from build123d import *

# Parameters (mm, degrees)
SKETCH1_W           = 250
SKETCH1_H           = 267.4
SKETCH1_R           = 2.5
SKETCH1_W_2         = 33
SKETCH1_H_2         = 90
BOSS_EXTRUDE1_DEPTH = 5
SKETCH6_W           = 250
SKETCH6_H           = 70.024397165
CUT_EXTRUDE4_DEPTH  = 6


with BuildPart() as part:
    # Sketch1 → Boss-Extrude1 (new body)
    with BuildSketch(Plane.XY):
        with Locations((-3272.432417868, -202.7)):
            Rectangle(SKETCH1_W, SKETCH1_H)
        with Locations((-3151.432417868, -193.5)):
            Circle(SKETCH1_R, mode=Mode.SUBTRACT)
        with Locations((-3151.432417868, -244.5)):
            Circle(SKETCH1_R, mode=Mode.SUBTRACT)
        with Locations((-3393.432417868, -244.5)):
            Circle(SKETCH1_R, mode=Mode.SUBTRACT)
        with Locations((-3393.432417868, -193.5)):
            Circle(SKETCH1_R, mode=Mode.SUBTRACT)
        with Locations((-3195.572417868, -219)):
            Rectangle(SKETCH1_W_2, SKETCH1_H_2, mode=Mode.SUBTRACT)
        with Locations((-3349.292417868, -219)):
            Rectangle(SKETCH1_W_2, SKETCH1_H_2, mode=Mode.SUBTRACT)
    extrude(amount=BOSS_EXTRUDE1_DEPTH)

    # Sketch6 → Cut-Extrude4 (cut, through all)
    with BuildSketch(Plane.XY.offset(5)):
        with BuildLine():
            Line((-3243.992329325, -69), (-3147.432417868, -69))
            Line((-3147.432417868, -69), (-3147.432417868, -182))
            Line((-3147.432417868, -182), (-3174.036756226, -182))
            Line((-3174.036756226, -182), (-3174.036756226, -154))
            Line((-3174.036756226, -154), (-3185.682810376, -154))
            ThreePointArc((-3185.682810376, -154), (-3237.221630697, -126.855339059), (-3243.992329325, -69))
        make_face()
        with Locations((-3272.432417868, -301.387801417)):
            Rectangle(SKETCH6_W, SKETCH6_H)
        with BuildLine():
            Line((-3300.872506412, -69), (-3397.432417868, -69))
            Line((-3397.432417868, -69), (-3397.432417868, -182))
            Line((-3397.432417868, -182), (-3370.82807951, -182))
            Line((-3370.82807951, -182), (-3370.82807951, -154))
            Line((-3370.82807951, -154), (-3359.18202536, -154))
            ThreePointArc((-3359.18202536, -154), (-3307.64320504, -126.855339059), (-3300.872506412, -69))
        make_face()
    extrude(amount=-CUT_EXTRUDE4_DEPTH, mode=Mode.SUBTRACT)


solid = part.part
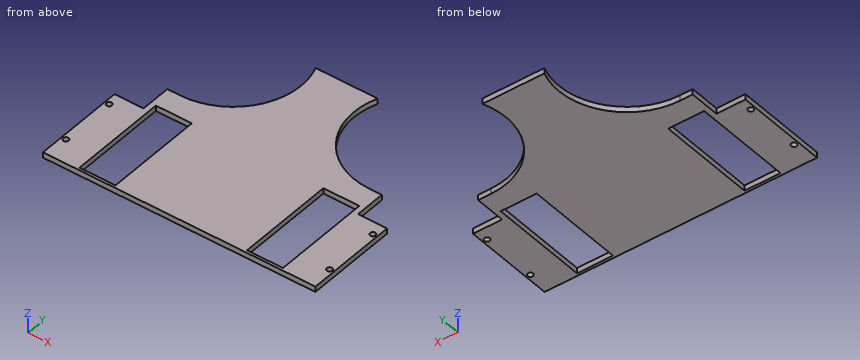
Input: part model. Units: mm. Frame: model coordinates. Round coordinates to 2 decimals unless told otherwise and drop trailing zeros. Order: outer loops, then holes, each group sorted by start corner. A loop starts at its lowest first (then second) coordinate and runs counter-clockwise, first axis right, second up.
1. Cut plane B-B, the plane z = 3.5. Output: boundary loops of the cut face in (x, y).
The answers:
outline: (-3397.43, -266.38) - (-3147.43, -266.38) - (-3147.43, -182) - (-3174.04, -182) - (-3174.04, -154) - (-3185.68, -154) arc R62.5 cw to (-3243.99, -69) - (-3300.87, -69) arc R62.5 cw to (-3359.18, -154) - (-3370.83, -154) - (-3370.83, -182) - (-3397.43, -182) - close; hole circle Ø5 at (-3393.43, -244.5); hole circle Ø5 at (-3393.43, -193.5); hole (-3365.79, -264) - (-3332.79, -264) - (-3332.79, -174) - (-3365.79, -174) - close; hole (-3212.07, -264) - (-3179.07, -264) - (-3179.07, -174) - (-3212.07, -174) - close; hole circle Ø5 at (-3151.43, -244.5); hole circle Ø5 at (-3151.43, -193.5)
2. Material intervals for line 1 (X direction, y = -178.5, z = 2.8); line 2 (X direction, y = -244.5, z = 3.7); line 3 (X direction, y = -201.5, z = 3.15), sorted ascending.
The answers:
line 1: x = -3370.83 to -3365.79, -3332.79 to -3212.07, -3179.07 to -3174.04
line 2: x = -3397.43 to -3395.93, -3390.93 to -3365.79, -3332.79 to -3212.07, -3179.07 to -3153.93, -3148.93 to -3147.43
line 3: x = -3397.43 to -3365.79, -3332.79 to -3212.07, -3179.07 to -3147.43
3. Cut plane A-A, the plane y = -177. Output: boundary loops of the cut face in (x, z).
The answers:
outline: (-3370.83, 0) - (-3365.79, 0) - (-3365.79, 5) - (-3370.83, 5) - close; (-3332.79, 0) - (-3212.07, 0) - (-3212.07, 5) - (-3332.79, 5) - close; (-3179.07, 0) - (-3174.04, 0) - (-3174.04, 5) - (-3179.07, 5) - close
4. Cut plane C-C, the plane y = -252. Output: boundary loops of the cut face in (x, z).
The answers:
outline: (-3397.43, 0) - (-3365.79, 0) - (-3365.79, 5) - (-3397.43, 5) - close; (-3332.79, 0) - (-3212.07, 0) - (-3212.07, 5) - (-3332.79, 5) - close; (-3179.07, 0) - (-3147.43, 0) - (-3147.43, 5) - (-3179.07, 5) - close
5. Pin query (flat end, axial travel): P1, Ø2.5, axis at x = -3349.5, z = 2, coming from the +Y side; P2, Ø1, axis at x = -3177, z = 1, coming from the +Y side. Return the tip coordinate at first contact, or that it passes through.
The answers:
P1: stops at y = -153.04
P2: stops at y = -154
6. Cut plane D-D, the plane x = -3167. Output: boundary loops of the cut face in (y, z), then the cut area to 3 significant figures.
The answers:
outline: (-266.38, 0) - (-182, 0) - (-182, 5) - (-266.38, 5) - close
area: 422 mm2
